For this review, take the finished solid that the model builds, in its own axes (mm). A direction names the side the tool comes from. Coordinates: 2 decimals unless noted, no trailing zeros. Write each loop counter-clockwise with the first axis right and the second up, starting at its lowest first coordinate (ties: lowest second). Pieces come first, ordered by that corner, then holes. Notation, with made-up numbers: (50, -5.75) -> (100, -5.75) arc R30 cw to (100, 26.25) -> close; hole circle Ø1 at (15, 30). An arc over 180 degrees is marked (long way). One line per item, written item: value. Start each with the question number.
1) Add section C-C (y = 9.5). State the section outline as (x, z) points (1 decimal), and give its area (3 significant figures).
2) For pin 1 Ø1.5 at (y, z) = (-31, 1) entering from +X; pin 2 Ø1 at (y, z) = (-13, 1.5) entering from +X, all flat-tipped, find the tip position at first contact; note any pin that passes through.
3) Mouldability with a two-part tool opening along Y and no side actions: class faces 1 (the flat face through (-7, -51.962, 2)), 2 (the cylindrical face through (9.02, 10.17, 1.57)), 3 (the cylindrical face through (3.613, -58.516, 1.61)), 4 (the flat face through (0, 31.785, 2)) as released by +Y, released by -Y, zero draft, split by the parting line, or undercut.
4) Machinability: for faces 5 (the flat face through (-28.09, 28.47, 1.57)), 6 (the cylindrical face through (-3.01, 22.35, 1.57)), 7 (the flat face through (25.46, 28.35, 1.57)), which of the approach directions +Z, -Z, +X, -X, +Y, -Y give a long, thin tool a straight path to every point of the face, cutting with its end or side? Answer none if there is none.
5) Add section B-B (y = -12). State the section outline as (x, z) points (3 decimals).
6) Add section A-A (x = 17). State the section outline as (y, z) points (3 decimals), and give its area (3 significant figures).
7) For probe 1 along Y at (x, z) = (0, 1.8); probe 2 along Y at (x, z) = (10.5, 1.2); probe 3 along X at (y, z) = (-47.5, 1.95), list the stretches that pass through material, from the lowest coordinate up. Write a range as from..to.
from build123d import *

# Parameters (mm, degrees)
F2_DEPTH  = 3.175
F1_R      = 13.594235125
F4_DEPTH  = 3.175
F6_DEPTH  = 3.175
F7_R      = 1.27
F8_R      = 0.762
F9_R      = 0.79375
F10_DEPTH = 3.176
F11_R     = 2.54


with BuildPart() as f2:
    # F1 (on face) → F2 (new body)
    with BuildSketch(Plane.XY):
        with BuildLine():
            Line((31.4070041795, 31.7847206253), (-31.4070041795, 31.7847206253))
            Line((-31.4070041795, 31.7847206253), (-26.3270041795, 26.7047206253))
            ThreePointArc((-26.3270041795, 26.7047206253), (-29.4018182362, -17.3120874939), (-6.8377400748, -55.230371411))
            Line((-6.8377400748, -55.230371411), (-2.5995985028, -50.5016658783))
            ThreePointArc((-2.5995985028, -50.5016658783), (-19.1698848855, -13.2713854087), (0, 22.6894778752))
            ThreePointArc((0, 22.6894778752), (20.2259208041, -17.2835334321), (2.6025941293, -58.4702772006))
            Line((2.6025941293, -58.4702772006), (6.8377400748, -63.2016658783))
            ThreePointArc((6.8377400748, -63.2016658783), (30.2976275511, -20.9804187613), (22.6081860771, 26.7047206253))
            Line((22.6081860771, 26.7047206253), (31.4070041795, 31.7847206253))
        make_face()
    extrude(amount=F2_DEPTH)



with BuildPart() as f2b:
    # F1 (on face) → F2, piece 2 (new body)
    with BuildSketch(Plane.XY):
        Circle(F1_R)
    extrude(amount=F2_DEPTH)


with BuildPart() as f2_1:
    add(f2.part)

    add(f2b.part)  # F4 merges F2b
    # F3 (on face) → F4 (join, through all)
    with BuildSketch(Plane.XY):
        with BuildLine():
            Line((-5.2498336251, 24.2303351167), (-13.4892699034, 7.3891431238))
            ThreePointArc((-13.4892699034, 7.3891431238), (-7.7433725843, -12.2768772355), (11.922647775, -6.5309799163))
            Line((11.922647775, -6.5309799163), (9.7925756653, -5.3641704599))
            ThreePointArc((9.7925756653, -5.3641704599), (-7.8384100149, 2.474239555), (0, 20.1052252351))
            Line((0, 20.1052252351), (-5.2498336251, 24.2303351167))
        make_face()
    extrude(amount=F4_DEPTH)

    # F5 (on face) → F6 (cut, through all)
    with BuildSketch(Plane.XY):
        Polygon((-3.9079916846, -49.3622544157), (-3.9079916846, -51.9615052849), (-10.2579916846, -51.9615052849), (-10.2579916846, -62.6840499783), (0, -56.9217726588), (-2.6145169004, -45.902473209), align=None)
        with BuildLine():
            Line((0, 19.5056907833), (0, 22.6894778752))
            ThreePointArc((0, 22.6894778752), (-2.5244121089, 24.0453912744), (-5.359141473, 24.4642791758))
            Line((-5.359141473, 24.4642791758), (-5.1168514161, 22.9205221383))
            ThreePointArc((-5.1168514161, 22.9205221383), (-3.237454866, 22.4415366371), (-1.5200501793, 21.5403820193))
            Line((-1.5200501793, 21.5403820193), (0, 19.5056907833))
        make_face()
    extrude(amount=F6_DEPTH, mode=Mode.SUBTRACT)

    # F7
    f7_edges = [f2_1.edges().sort_by_distance(p)[0] for p in [
        (-31.407004, 31.784721, 1.5875),
        (-26.327004, 26.704721, 1.5875),
        (31.407004, 31.784721, 1.5875),
        (22.608186, 26.704721, 1.5875),
        (-3.907992, -49.362254, 1.5875),
        (-3.907992, -51.961505, 1.5875),
        (-10.257992, -51.961505, 1.5875),
    ]]
    fillet(f7_edges, radius=F7_R)

    # F8
    f8_edges = [f2_1.edges().sort_by_distance(p)[0] for p in [
        (-5.359141, 24.464279, 1.5875),
        (-5.116851, 22.920522, 1.5875),
    ]]
    fillet(f8_edges, radius=F8_R)

    # F9 (on face) → F10 (cut, through all)
    with BuildSketch(Plane.XY.offset(3.175)):
        with Locations((0, -0.2915779182)):
            Circle(F9_R)
    extrude(amount=-F10_DEPTH, mode=Mode.SUBTRACT)

    # F11
    f11_edges = [f2_1.edges().sort_by_distance(p)[0] for p in [
        (2.602594, -58.470277, 1.5875),
        (6.83774, -63.201666, 1.5875),
    ]]
    fillet(f11_edges, radius=F11_R)


solid = f2_1.part
Numbers:
1. outline: (-30.8, 0) -> (9.7, 0) -> (9.7, 3.2) -> (-30.8, 3.2) -> close; (11.9, 0) -> (29.2, 0) -> (29.2, 3.2) -> (11.9, 3.2) -> close
1. area: 183 mm²
2. pin 1: x = 28.05
2. pin 2: x = 31.28
3. face 1: released by -Y
3. face 2: undercut
3. face 3: undercut
3. face 4: released by +Y
4. face 5: +Z, -Z, -X
4. face 6: +Z, -Z
4. face 7: +Z, -Z, +X
5. outline: (-30.461, 0) -> (-19.107, 0) -> (-19.107, 3.175) -> (-30.461, 3.175) -> close; (-8.227, 0) -> (6.66, 0) -> (6.66, 3.175) -> (-8.227, 3.175) -> close; (19.791, 0) -> (31.311, 0) -> (31.311, 3.175) -> (19.791, 3.175) -> close
6. outline: (-52.031, 0) -> (-37.264, 0) -> (-37.264, 3.175) -> (-52.031, 3.175) -> close; (-0.7, 0) -> (31.785, 0) -> (31.785, 3.175) -> (-0.7, 3.175) -> close
6. area: 150 mm²
7. probe 1: -14.04..-1.09, 0.5..13.59, 22.69..31.78
7. probe 2: -59.69..-49.62, -8.66..8.63, 11.66..31.78
7. probe 3: -14.29..-5.85, 11.93..20.09
